Could you check a few things on this model? Use its own coordinates, in mm. A direction names the side the tool comes from. Give positions to 0.01 mm unless a question says otherwise; leave off trailing zeros. Loops run counter-clockwise (first coordinate to the right, second up) from the corner with the lowest first, then second, coordinate; pieces in that order, holes last. Notation, with made-up numbers: (47.25, 49.25) -> (86.25, 49.25) arc R8 cw to (86.25, 53.25) -> close; hole circle Ø11 at (-25.5, 23.25). An arc over 180 degrees is marked (long way). Write each question's results on one line, items separated by ' | '. Start each with the question number.
Q1. We'd pull the mould along Z, two halves only. Please class faces 3 (the face through (311, 8, 0)), 4 (the face through (630, 14, 7)), 5 (the face through (311, 13.8, 7)): released by +Z, released by -Z, zero draft, split by the parting line, or undercut.
Q2. If we section it at A-A, the plane y = 7: List the corners of the cut face in (x, z) for me, plus the area to 3 significant figures.
Q3. Which directions (+Z, -Z, +X, -X, +Y, -Y) give clear straight access to the entire face, cutting with the end or side of a thin tool? Please do faces 1 (the face through (311, 7, 13.8)), 2 (the face through (311, 15, 7)).
Q4. If I drill on line 1 along X through (y, z) = (0.35, 7.5); line 2 along Y through (x, z) = (495.5, 11), over which ranges is the centre line in solid material (lowest first)?
Q5. If we section it at B-B, the plane x = 416: List the corners of the cut face in (y, z) for me.
from build123d import *

# Parameters (mm, degrees)
SKETCH_1_W          = 630
SKETCH_1_H          = 15
EXTRUDE_1_DEPTH     = 15
SKETCH_2_R          = 1.5
CUT_EXTRUDE_1_DEPTH = 631.357041684
SKETCH_3_W          = 12.6
SKETCH_3_H          = 12.6
CUT_EXTRUDE_2_DEPTH = 631.357041684


with BuildPart() as part:
    # ｽｹｯﾁ1 → ﾎﾞｽ - 押し出し1 (new body)
    with BuildSketch(Plane.XY):
        with Locations((315, 7.5)):
            Rectangle(SKETCH_1_W, SKETCH_1_H)
    extrude(amount=EXTRUDE_1_DEPTH)

    # ｽｹｯﾁ2 → ｶｯﾄ - 押し出し1 (cut, through all)
    with BuildSketch(Plane(origin=(0, 15, 0), x_dir=(1, 0, 0), z_dir=(0, 1, 0))):
        with Locations(Location((6, -7.5, 0), (0, 0, 270))):
            Circle(SKETCH_2_R)
        with Locations(Location((624, -7.5, 0), (0, 0, 270))):
            Circle(SKETCH_2_R)
    extrude(amount=-CUT_EXTRUDE_1_DEPTH, mode=Mode.SUBTRACT)

    # ｽｹｯﾁ3 → ｶｯﾄ - 押し出し2 (cut, through all)
    with BuildSketch(Plane.ZY):
        with Locations((7.5, 7.5)):
            Rectangle(SKETCH_3_W, SKETCH_3_H)
    extrude(amount=-CUT_EXTRUDE_2_DEPTH, mode=Mode.SUBTRACT)


solid = part.part
Final values:
1) face 3: released by -Z | face 4: zero draft | face 5: undercut
2) outline: (0, 0) -> (630, 0) -> (630, 1.2) -> (0, 1.2) -> close; (0, 13.8) -> (630, 13.8) -> (630, 15) -> (0, 15) -> close | area: 1,510 mm²
3) face 1: +X, -X | face 2: +Z, -Z, +X, -X, +Y
4) line 1: x = 0 to 4.5, 7.5 to 622.5, 625.5 to 630 | line 2: y = 0 to 1.2, 13.8 to 15
5) outline: (0, 0) -> (15, 0) -> (15, 15) -> (0, 15) -> close; hole (1.2, 1.2) -> (13.8, 1.2) -> (13.8, 13.8) -> (1.2, 13.8) -> close
